Can you work these out from the model? Positions are in its coordinate system, mm. A direction names the side the tool comes from. Round coordinates to 2 decimals unless told otherwise and drop trailing zeros. Write each loop counter-clockwise with the first axis right and the second up, starting at its lowest first coordinate (ties: lowest second). Pieces come first, ordered by that corner, then holes. Notation, with made-up numbers: (42, -7.5) -> (63, -7.5) arc R14 cw to (63, 10.5) -> close; hole circle Ø5 at (56.5, -6). An arc over 180 degrees is marked (long way). Use CSV: the item, a comma, the result in double quotes.
Autodesk Fusion 360 part; units mm, degrees
sketch "Sketch1" plane through (0, 0, 0) normal (0, 0, 1) x (1, 0, 0)
  line L0 (0, 0) -> (53, 0)
  line L1 (53, 0) -> (53, 50)
  line L2 (53, 50) -> (0, 50)
  line L3 (0, 50) -> (0, 0)
  line L4 (12, 7.9) -> (42, 7.9)
  arc A0 (42, 7.9) -> (42, 12.1) centre (42, 10) ccw
  line L5 (42, 12.1) -> (12, 12.1)
  arc A1 (12, 12.1) -> (12, 7.9) centre (12, 10) ccw
  line L6 (12, 10) -> (42, 10) construction
  line L7 (0, 25) -> (53, 25) construction
  line L8 (42, 37.9) -> (12, 37.9)
  arc A2 (12, 42.1) -> (12, 37.9) centre (12, 40) ccw
  line L9 (12, 42.1) -> (42, 42.1)
  arc A3 (42, 37.9) -> (42, 42.1) centre (42, 40) ccw
  line L10 (49.4724, 50) -> (53.0079, 46.4645)
  line L11 (49.4724, 50) -> (52.8478, 50) construction
  line L12 (49.4724, 0) -> (53.0079, 3.5355)
  line L13 (0, 50) -> (2, 50)
  line L14 (2, 50) -> (2, 0)
  line L15 (2, 0) -> (0, 0)
  line L16 (0, 0) -> (0, 50)
  dimension "d1" = 53
  dimension "d2" = 50
  dimension "d3" = 4.2
  dimension "d4" = 11
  dimension "d5" = 10
  dimension "d6" = 30
  dimension "d9" = 45
  dimension "d10" = 5
extrude "Extrude1" add sketch "Sketch1" against normal blind 2 contours L0 L2 L3 L13 L14 L15 L16 | L0 L1 L2 L10 L12 L14
extrude "Extrude2" add sketch "Sketch1" along normal blind 49 contours L0 L2 L3 L13 L14 L15 L16
sketch "Sketch2" plane through (0, 0, 0) normal (-1, 0, 0) x (0, -1, 0)
  line L0 (-50, 49) -> (-50, -2)
  line L1 (-50, -2) -> (0, -2)
  line L2 (0, -2) -> (0, 49)
  line L3 (0, 49) -> (-50, 49)
  circle A0 centre (-25, 23.5) radius 11.05
  line L4 (-40.5, 39) -> (-9.5, 39) construction
  line L5 (-9.5, 39) -> (-9.5, 8) construction
  line L6 (-9.5, 8) -> (-40.5, 8) construction
  line L7 (-40.5, 8) -> (-40.5, 39) construction
  line L8 (-40.5, 39) -> (-9.5, 8) construction
  line L9 (-9.5, 39) -> (-40.5, 8) construction
  circle A1 centre (-40.5, 39) radius 1.75
  circle A2 centre (-9.5, 39) radius 1.75
  circle A3 centre (-40.5, 8) radius 1.75
  circle A4 centre (-9.5, 8) radius 1.75
  line L10 (-50, 45.4997) -> (-46.4645, 49.0353)
  line L11 (-50, 45.4997) -> (-45, 45.4997) construction
  line L12 (-25, 49) -> (-25, -2)
  line L13 (0, 45.4997) -> (-3.5355, 49.0353)
  point P0 (-25, 23.5)
  dimension "d13" = 22.1
  dimension "d14" = 31
  dimension "d15" = 31
  dimension "d16" = 3.5
  dimension "d17" = 3.5
  dimension "d18" = 3.5
  dimension "d19" = 3.5
  dimension "d20" = 45
  dimension "d21" = 5
extrude "Extrude3" cut sketch "Sketch2" against normal blind 2 contours L0 L3 L10 | L2 L3 L13 | A0 L12 | A0 L12 | A1 | A2 | A3 | A4
sketch "Sketch3" plane through (0, 0, 0) normal (0, -1, 0) x (1, 0, 0)
  line L0 (2, 45.4997) -> (0, 45.4997)
  line L1 (0, 45.4997) -> (0, -2)
  line L2 (0, -2) -> (49.4724, -2)
  line L3 (49.4724, -2) -> (49.4724, 0)
  line L4 (49.4724, 0) -> (2, 0)
  line L5 (2, 0) -> (2, 45.4997)
  line L6 (2, 0) -> (2, 20) construction
  line L7 (2, 0) -> (15, 0) construction
  line L8 (2, 20) -> (15, 0)
  dimension "d24" = 20
  dimension "d25" = 13
extrude "Extrude4" add sketch "Sketch3" against normal blind 2 contours L4 L5 L8
ref_plane "WorkPlane1" through (24.7362, 25, 21.7499) normal (0, -1, 0) x (-1, 0, 0)
mirror "Mirror1" about plane through (24.7362, 25, 21.7499) normal (0, -1, 0) of "Extrude4"
Q1. Suppose I cut it at D-D (z = 5). Write out the boundary of the cut face in (x, y).
Resolved:
outline,"(0, 0) -> (11.75, 0) -> (11.75, 2) -> (2, 2) -> (2, 48) -> (11.75, 48) -> (11.75, 50) -> (0, 50) -> close"
Q2. On a 3-axis mill with a long thin cutter (end or side, diameter ignored), from which of +Z, -Z, +X, -X, +Y, -Y can I reach the whole of each face in a straight line? I mean faces 1 (the face through (27, 7.9, -1)), 2 (the face through (8, 50, 10)), 3 (the face through (27, 25, 0)). Say none if no direction works.
Resolved:
face 1,"+Z, -Z"
face 2,"+Z, -Z, +X, -X, +Y"
face 3,"+Z, +X"
Q3. Please list where these lines run through material, in increasing order: probe 1 along Z at (x, y) = (1, 40.5); probe 2 along Z at (x, y) = (0.9, 25); probe 3 along Z at (x, y) = (18.5, 24.5).
Resolved:
probe 1,"z = -2 to 6.25, 9.75 to 37.25, 40.75 to 49"
probe 2,"z = -2 to 12.45, 34.55 to 49"
probe 3,"z = -2 to 0"
Q4. Suppose I cut it at A-A (z = 39). Write out the boundary of the cut face in (x, y), and give its area (3 significant figures).
Resolved:
outline,"(0, 0) -> (2, 0) -> (2, 7.75) -> (0, 7.75) -> close; (0, 11.25) -> (2, 11.25) -> (2, 38.75) -> (0, 38.75) -> close; (0, 42.25) -> (2, 42.25) -> (2, 50) -> (0, 50) -> close"
area,"86.0 mm^2"
Q5. If we mould it in two halves opening along Z, with no side actions, what happens to faces 4 (the face through (9.9, 10, -1)), 5 (the face through (8.41, 0.99, 10.14)), 6 (the face through (0.99, 9.88, 37.29))? For each: released by +Z, released by -Z, zero draft, split by the parting line, or undercut.
Resolved:
face 4,"zero draft"
face 5,"released by +Z"
face 6,"undercut"
Q6. Suppose I cut it at C-C (y = 25). Write out the boundary of the cut face in (x, z), and give its area (3 significant figures).
Resolved:
outline,"(0, -2) -> (53, -2) -> (53, 0) -> (2, 0) -> (2, 12.45) -> (0, 12.45) -> close; (0, 34.55) -> (2, 34.55) -> (2, 49) -> (0, 49) -> close"
area,"160 mm^2"
Q7. Will these pins go through, and if not, where does the flat tip stop? P1, Ø3, axis at y = 26, z = 31, coming from the -X side; P2, Ø12, axis at y = 35, z = 30.5, coming from the +X side; P3, Ø12, axis at x = 24.5, y = 24.5, coming from the +Z side.
Resolved:
P1,"passes through"
P2,"stops at x = 2"
P3,"stops at z = 0"
Q8. Suppose I cut it at B-B (x = 39). Write out the boundary of the cut face in (y, z).
Resolved:
outline,"(0, -2) -> (7.9, -2) -> (7.9, 0) -> (0, 0) -> close; (12.1, -2) -> (37.9, -2) -> (37.9, 0) -> (12.1, 0) -> close; (42.1, -2) -> (50, -2) -> (50, 0) -> (42.1, 0) -> close"
